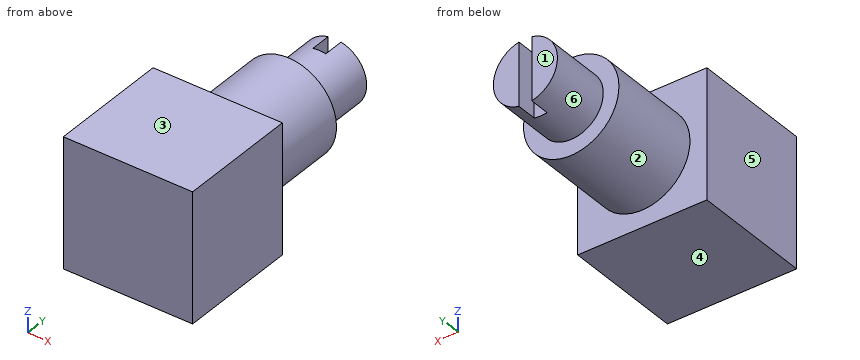
```python
from build123d import *

# Parameters (mm, degrees)
SKETCH1_W               = 12.6
SKETCH1_H               = 12.6
BOSS_EXTRUDE1_DEPTH     = 11.75
SKETCH2_R               = 4.65
BOSS_EXTRUDE2_DEPTH     = 9.3
SKETCH3_R               = 3.125
BOSS_EXTRUDE3_DEPTH     = 6
CUT_EXTRUDE1_DEPTH      = 29.479510178
CUT_EXTRUDE1_DEPTH_BACK = 29.479510178
SKETCH4_W               = 1.25
SKETCH4_H               = 2


with BuildPart() as part:
    # Sketch1 → Boss-Extrude1 (new body)
    with BuildSketch(Plane(origin=(0, 0, 0), x_dir=(1, 0, 0), z_dir=(0, 1, 0))):
        Rectangle(SKETCH1_W, SKETCH1_H)
    extrude(amount=BOSS_EXTRUDE1_DEPTH)

    # Sketch2 → Boss-Extrude2 (add)
    with BuildSketch(Plane(origin=(0, 11.75, 0), x_dir=(1, 0, 0), z_dir=(0, 1, 0))):
        with Locations(Location((0, 0, 0), (0, 0, 270))):
            Circle(SKETCH2_R)
    extrude(amount=BOSS_EXTRUDE2_DEPTH)

    # Sketch3 → Boss-Extrude3 (add)
    with BuildSketch(Plane(origin=(0, 21.05, 0), x_dir=(1, 0, 0), z_dir=(0, 1, 0))):
        with Locations(Location((0, 0, 0), (0, 0, 270))):
            Circle(SKETCH3_R)
    extrude(amount=BOSS_EXTRUDE3_DEPTH)

    # Sketch4 → Cut-Extrude1 (cut, two sides: drawn at the far end of the back side and taken through both)
    with BuildSketch(Plane.XY.offset(-CUT_EXTRUDE1_DEPTH_BACK)):
        with Locations((0, 26.05)):
            Rectangle(SKETCH4_W, SKETCH4_H)
    extrude(amount=CUT_EXTRUDE1_DEPTH + CUT_EXTRUDE1_DEPTH_BACK, mode=Mode.SUBTRACT)


solid = part.part
```
Input: part model. Units: mm. Frame: model coordinates. Face numbers are marked on the shaded views. A direction names the side the tool comes from. Coordinates: 2 decimals unless noted, no trailing zeros. Write each loop counter-clockwise with the first axis right and the second up, starting at its lowest first coordinate (ties: lowest second). Pieces come first, ordered by that corner, then holes. Notation, with made-up numbers: (-19.5, 11) - (13.5, 11) arc R15 cw to (13.5, 18) - close; hole circle Ø10 at (10.5, -3). An arc over 180 degrees is marked (long way). Put each result on its own line as item: value. Start each with the question number.
1) Cut plane A-A (x = 0). Return the cut outline in (y, z) (3 decimals).
2) Cut plane C-C (y = 19). Return the cut outline in (x, z).
3) Ray query, L1, parallel to Y at x = 4, z = 2.5; L2, parallel to Z at x = 0, y = 22.25 (3 decimals); L3, parallel to Y at x = 3.5, z = -3. Return the intervals inside material, ascending.
4) Cut plane D-D (x = 2.5). Return the cut outline in (y, z) (3 decimals), plus the area to 3 significant figures.
5) Reachability of the marked faces 1 and 2 from +Z, -Z, +X, -X, +Y, -Y: full face, straight path, thin tool, end or side. Return the list, or none.
6) Contact query for flat-ended pins moving along their axis: pin 1 (6 mm diameter, centred on y = 16, z = 5, fed in from +X); pin 2 (2 mm diameter, centred on y = 26, z = -0.5, fed in from -X) (3 decimals); pin 3 (1 mm diameter, centred on x = 0, z = -0.5, fed in from +Y). Output: stop coordinate, or through.
7) Mould query, pull axis Z, two halves, no side actions, for the marked faces 3, 4, 5 and 6. Classes: pulls with the +Z half, pulls with the -Z half, needs draft (parallel to the pull), parting line crosses it, or undercut.
8) Cut plane B-B (z = -5). Return the cut outline in (x, y).
Resolved:
1. outline: (0, -6.3) - (11.75, -6.3) - (11.75, -4.65) - (21.05, -4.65) - (21.05, -3.125) - (25.05, -3.125) - (25.05, 3.125) - (21.05, 3.125) - (21.05, 4.65) - (11.75, 4.65) - (11.75, 6.3) - (0, 6.3) - close
2. outline: circle Ø9.3 at (0, 0)
3. L1: y = 0 to 11.75
3. L2: z = -3.125 to 3.125
3. L3: y = 0 to 21.05
4. outline: (0, -6.3) - (11.75, -6.3) - (11.75, -3.921) - (21.05, -3.921) - (21.05, -1.875) - (27.05, -1.875) - (27.05, 1.875) - (21.05, 1.875) - (21.05, 3.921) - (11.75, 3.921) - (11.75, 6.3) - (0, 6.3) - close
4. area: 243 mm2
5. face 1: +Z, -Z, +X, -X, +Y
5. face 2: +Y
6. pin 1: stops at x = 4.2
6. pin 2: stops at x = -3.125
6. pin 3: stops at y = 25.05
7. face 3: pulls with the +Z half
7. face 4: pulls with the -Z half
7. face 5: needs draft
7. face 6: parting line crosses it
8. outline: (-6.3, 0) - (6.3, 0) - (6.3, 11.75) - (-6.3, 11.75) - close
